```python
from build123d import *

# Parameters (mm, degrees)
F_70X45X5_1_DEPTH   = 2180
CUT_EXTRUDE_1_REACH = 2202.858
SKETCH_12_R         = 7
CUT_EXTRUDE_2_REACH = 2202.858
SKETCH_13_R         = 7
CHAMFER_1_SIZE      = 30
CHAMFER_2_SIZE      = 30


with BuildPart() as part:
    # 草图11 → 不等边角钢 70X45X5(1) (new body)
    with BuildSketch(Plane(origin=(1090, 1887.93538025, 0), x_dir=(0.86602540378444, -0.4999999999999978, 0), z_dir=(-0.4999999999999978, -0.86602540378444, 0))):
        with BuildLine():
            Line((0, 70), (0, 0))
            Line((0, 0), (45, 0))
            Line((45, 0), (45, 3.33))
            ThreePointArc((45, 3.33), (44.510868325, 4.510868325), (43.33, 5))
            Line((43.33, 5), (12.5, 5))
            ThreePointArc((12.5, 5), (7.196699141, 7.196699141), (5, 12.5))
            Line((5, 12.5), (5, 68.33))
            ThreePointArc((5, 68.33), (4.510868325, 69.510868325), (3.33, 70))
            Line((3.33, 70), (0, 70))
        make_face()
    extrude(amount=F_70X45X5_1_DEPTH)

    # 草图12 → 切除-拉伸1 (cut, up to next)
    with BuildSketch(Plane(origin=(0, 0, 0), x_dir=(0, 0, 1), z_dir=(-0.86602540378444, 0.49999999999999784, 0)), mode=Mode.PRIVATE) as cut_extrude_1_sk1:
        with Locations(Location((40, 30, 0), (0, 0, 270))):
            Circle(SKETCH_12_R)
    cut_extrude_1_tool1 = extrude(cut_extrude_1_sk1.sketch, amount=-CUT_EXTRUDE_1_REACH, mode=Mode.PRIVATE) & part.part
    # 草图12 → 切除-拉伸1 (cut, up to next)
    with BuildSketch(Plane(origin=(0, 0, 0), x_dir=(0, 0, 1), z_dir=(-0.86602540378444, 0.49999999999999784, 0)), mode=Mode.PRIVATE) as cut_extrude_1_sk2:
        with Locations(Location((40, 110, 0), (0, 0, 270))):
            Circle(SKETCH_12_R)
    cut_extrude_1_tool2 = extrude(cut_extrude_1_sk2.sketch, amount=-CUT_EXTRUDE_1_REACH, mode=Mode.PRIVATE) & part.part
    add(cut_extrude_1_tool1.solids().sort_by_distance((15, 25.980762, 40))[0], mode=Mode.SUBTRACT)
    add(cut_extrude_1_tool2.solids().sort_by_distance((55, 95.262794, 40))[0], mode=Mode.SUBTRACT)

    # 草图13 → 切除-拉伸2 (cut, up to next)
    with BuildSketch(Plane(origin=(0, 0, 0), x_dir=(0, 0, 1), z_dir=(-0.86602540378444, 0.49999999999999784, 0)), mode=Mode.PRIVATE) as cut_extrude_2_sk1:
        with Locations(Location((40.004723234, 2070, 0), (0, 0, 270))):
            Circle(SKETCH_13_R)
    cut_extrude_2_tool1 = extrude(cut_extrude_2_sk1.sketch, amount=-CUT_EXTRUDE_2_REACH, mode=Mode.PRIVATE) & part.part
    # 草图13 → 切除-拉伸2 (cut, up to next)
    with BuildSketch(Plane(origin=(0, 0, 0), x_dir=(0, 0, 1), z_dir=(-0.86602540378444, 0.49999999999999784, 0)), mode=Mode.PRIVATE) as cut_extrude_2_sk2:
        with Locations(Location((40.004723234, 2150, 0), (0, 0, 270))):
            Circle(SKETCH_13_R)
    cut_extrude_2_tool2 = extrude(cut_extrude_2_sk2.sketch, amount=-CUT_EXTRUDE_2_REACH, mode=Mode.PRIVATE) & part.part
    add(cut_extrude_2_tool1.solids().sort_by_distance((1035, 1792.672586, 40.004723))[0], mode=Mode.SUBTRACT)
    add(cut_extrude_2_tool2.solids().sort_by_distance((1075, 1861.954618, 40.004723))[0], mode=Mode.SUBTRACT)

    # 倒角1
    # the kernel refuses this chamfer: 30 mm, written as the material it takes off along each edge
    with BuildSketch(Plane(origin=(1159.698148536, 1847.695135431, 70), x_dir=(-0.4998109584556461, -0.8656979742248816, 0.027495876610586955), z_dir=(-0.86602540378444, 0.4999999999999978, 0))) as chamfer_1_piece_1:
        Polygon((CHAMFER_1_SIZE * 0.999621916911, -CHAMFER_1_SIZE * 0.0274958766106), (-CHAMFER_1_SIZE * 0.0274958766106, -CHAMFER_1_SIZE * 0.999621916911), (0, 0), align=None)
    extrude(amount=157.630979278, mode=Mode.SUBTRACT)

    # 倒角2
    # the kernel refuses this chamfer: 30 mm, written as the material it takes off along each edge
    with BuildSketch(Plane(origin=(69.698148536, -40.240244819, 70), x_dir=(-0.013747938305293052, -0.02381212764409008, -0.9996219169112966), z_dir=(-0.86602540378444, 0.4999999999999978, 0))) as chamfer_2_piece_1:
        Polygon((CHAMFER_2_SIZE * 0.999621916911, -CHAMFER_2_SIZE * 0.0274958766106), (-CHAMFER_2_SIZE * 0.0274958766106, -CHAMFER_2_SIZE * 0.999621916911), (0, 0), align=None)
    extrude(amount=157.630979278, mode=Mode.SUBTRACT)


solid = part.part
```
Source: CAD feature listing. Evaluate the final solid. Frame: model axes, mm. A direction names the side the tool comes from. Give positions to 0.01 mm unless a question says otherwise; leave off trailing zeros. Use a Markdown table: item, result.
Q1. Material intervals for line 1 (Z direction, x = 97, y = 99); line 2 (Y direction, x = 958, z = 44); line 3 (X direction, y = 1670.5, z = 30.5), sorted ascending. Write a range as [from, to].
A:
| item | result |
|---|---|
| line 1 | [0, 5] |
| line 2 | [1649.3, 1659.3] |
| line 3 | [964.46, 970.24] |
Q2. Access query for faces 1 (the face through (572, 946, 0)), 2 (the face through (556.96, 954.68, 40.02)). Directions: +Z, -Z, +X, -X, +Y, -Y. A direction counts if a zero-diameter tool reaches every point of the face in a straight line with its end or side. Return the directions, or none.
A:
| item | result |
|---|---|
| face 1 | -Z, +X, -X, +Y, -Y |
| face 2 | +Z, +X, -Y |
Q3. First-contact query: P1, Ø8, axis at x = 532.5, z = 25, coming from the -Y side; P2, Ø1, axis at y = 189.5, z = 61, coming from the -X side; P3, Ø1, axis at y = 1622.5, z = 21, coming from the -X side. Flat tips, straight axial feed; report the tip coordinate or a pass-through.
A:
| item | result |
|---|---|
| P1 | y = 905.39 |
| P2 | x = 109.12 |
| P3 | x = 936.46 |
